Verification items for this drawing (mm, ordinates from the low corner). A direction names the side the tool comes from. Round coordinates to 2 decimals unless told otherwise and drop trailing zeros. Order: outer loops, then holes, each group sorted by start corner. A loop starts at its lowest first (then second) coordinate and runs counter-clockwise, first axis right, second up. Notation, with made-up numbers: M -9,10 L 46,10 A20 ccw 46,18 Z; hole C 18,88.25 d8. An arc over 180 degrees is marked long. Return JSON: item names as keys, results as strings. Group by question number.
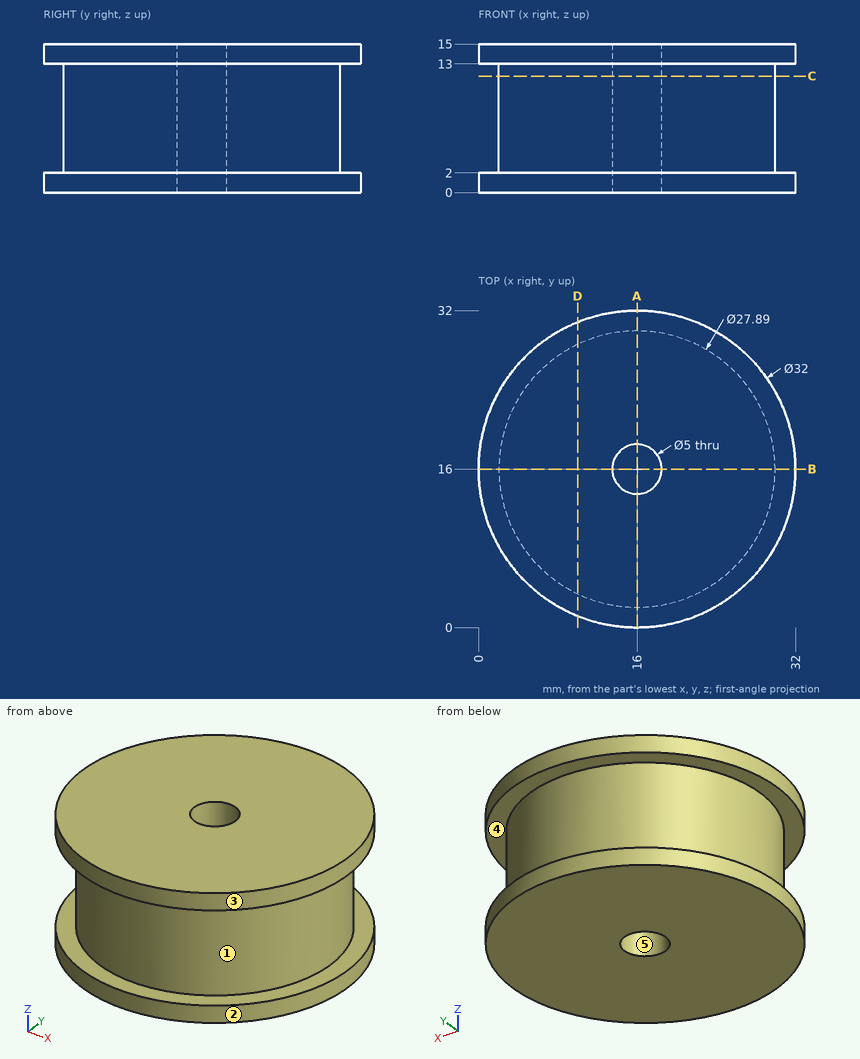
Q1. Section check A-A on x = 16. Record the cut outline in (y, z) (3 decimals), plus the area to 3 significant figures.
Q2. Section check D-D on x = 10. Record the cut outline in (y, z).
Q3. Release check for a two-part mould opening along Y. For the marked faces 3, 4 and 5 record: +Y half, -Y half, draft (parallel to the pull), parting line (faces both ways), or undercut.
Q4. Section check C-C on z = 11.75. Record the cut outline in (x, y) (3 decimals), plus the area to 3 significant figures.
Q5. Set-up check for the marked faces 1 and 2: record each of +Z, -Z, +X, -X, +Y, -Y from which the full face is reachable in a straight line by a thin tool's end or side.
Q6. Material ranges on line 1 along Y through (x, z) = (16, 3.5) (3 decimals); line 2 along Z through (x, y) = (24, 28.5); line 3 along Y through (x, z) = (12, 5), recorded low to high.
Q7. Depth check by flat-ended pin: pin 1 Ø1 at (x, z) = (14, 10) entering from +Y; pin 2 Ø6 at (x, y) = (3.5, 9.5) entering from -Z; pin 3 Ø8 at (y, z) = (25.5, 4) entering from -X; pin 4 Ø4 at (y, z) = (24, 5.5) entering from -X. Enter the tip coordinate at first touch or a pass-through.
Geometry check:
{
 "1": {"outline": "M 0,0 L 13.5,0 L 13.5,15 L 0,15 L 0,13 L 2.055,13 L 2.055,2 L 0,2 Z; M 18.5,0 L 32,0 L 32,2 L 29.945,2 L 29.945,13 L 32,13 L 32,15 L 18.5,15 Z", "area": "360 mm^2"},
 "2": {"outline": "M 1.17,0 L 30.83,0 L 30.83,2 L 28.59,2 L 28.59,13 L 30.83,13 L 30.83,15 L 1.17,15 L 1.17,13 L 3.41,13 L 3.41,2 L 1.17,2 Z"},
 "3": {"face 3": "parting line", "face 4": "draft", "face 5": "undercut"},
 "4": {"outline": "C 16,16 d27.89; hole C 16,16 d5", "area": "591 mm^2"},
 "5": {"face 1": "none", "face 2": "+Z, -Z"},
 "6": {"line 1": "y = 2.055 to 13.5, 18.5 to 29.945", "line 2": "z = 0 to 2, 13 to 15", "line 3": "y = 2.64 to 29.36"},
 "7": {"pin 1": "stops at y = 29.86", "pin 2": "stops at z = 0", "pin 3": "stops at x = 1.18", "pin 4": "stops at x = 3.41"}
}
